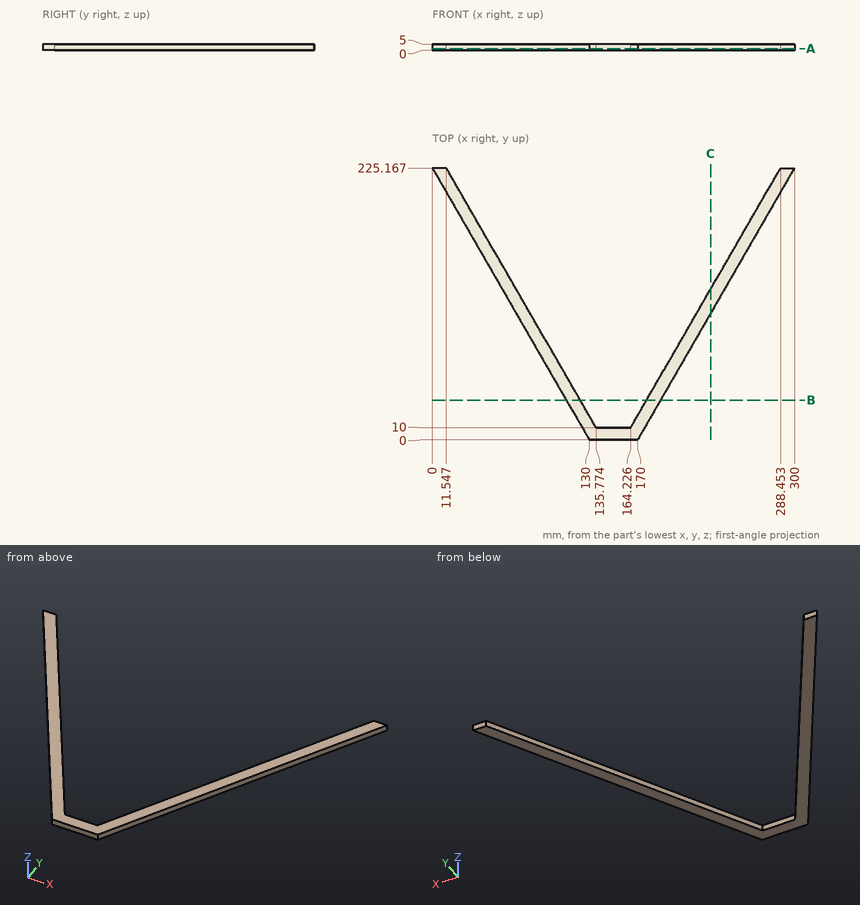
Print and shaded views of the part. All mm, measured from the part's lowest x, y and z. Coordinates: 2 decimals unless noted, no trailing zeros. Write each loop counter-clockwise with the first axis right and the second up, starting at its lowest first coordinate (ties: lowest second). Pieces come first, ordered by that corner, then holes. Notation, with made-up numbers: (45.5, 66.25) -> (95.5, 66.25) arc R22 cw to (95.5, 98.25) -> close; hole circle Ø11 at (17.25, 15). An arc over 180 degrees is marked (long way). Use CSV: the item, a comma, the result in double quotes. Start each with the question number.
Q1. Cut at B-B, the plane y = 33. List the corners of the cut face in (x, z) (1 decimal).
Q2. Cut at A-A, the plane z = 1.25. List the corners of the cut face in (x, y), then the cut area to 3 significant figures.
Q3. Flat gauge pins, fed straight in: pin 1 Ø1.5 at (x, z) = (207.5, 1) entering from +Y; pin 2 Ø3 at (x, z) = (111, 3.5) entering from +Y (1 decimal); pin 3 Ø1 at (y, z) = (55.5, 3.5) entering from -X. Where does each tip first touch, or does it go through?
Q4. Drill centre lines: probe 1 along X at (y, z) = (153, 4.5) (1 decimal); probe 2 along Y at (x, z) = (161, 0.85); probe 3 along X at (y, z) = (65, 1.3). Where is each one in solid material? Low to high.
Q5. Cut at C-C, the plane x = 230.5. List the corners of the cut face in (y, z).
Checked values:
1,outline,"(110.9, 0) -> (122.5, 0) -> (122.5, 5) -> (110.9, 5) -> close; (177.5, 0) -> (189.1, 0) -> (189.1, 5) -> (177.5, 5) -> close"
2,outline,"(0, 225.17) -> (130, 0) -> (170, 0) -> (300, 225.17) -> (288.45, 225.17) -> (164.23, 10) -> (135.77, 10) -> (11.55, 225.17) -> close"
2,area,"5,430 mm²"
3,pin 1,"stops at y = 86.25"
3,pin 2,"stops at y = 55.5"
3,pin 3,"stops at x = 97.67"
4,probe 1,"x = 41.7 to 53.2, 246.8 to 258.3"
4,probe 2,"y = 0 to 10"
4,probe 3,"x = 92.47 to 104.02, 195.98 to 207.53"
5,outline,"(104.79, 0) -> (124.79, 0) -> (124.79, 5) -> (104.79, 5) -> close"
